Can you work these out from the model? Positions are in its coordinate system, mm. A direction names the side the tool comes from. Round coordinates to 2 decimals unless told otherwise and drop trailing zeros. Loops run counter-clockwise (first coordinate to the right, second up) from the corner with the lowest first, then second, coordinate; pieces in that order, holes last. Notation, with made-up numbers: (76.25, 74.25) -> (116.25, 74.25) arc R26 ccw to (116.25, 111.25) -> close; hole circle Ø5 at (-9.75, -16.5). An arc over 180 degrees is marked (long way). Use a Markdown table: item, result.
Autodesk Inventor part; units mm, degrees
ref_plane "YZ Plane" through (0, 0, 0) normal (1, 0, 0) x (0, 1, 0)
ref_plane "XZ Plane" through (0, 0, 0) normal (0, 1, 0) x (-1, 0, 0)
ref_plane "XY Plane" through (0, 0, 0) normal (0, 0, 1) x (1, 0, 0)
sketch "Sketch1" plane through (0, 0, 0) normal (0, 0, 1) x (1, 0, 0)
  line L0 (0, -70) -> (15, -70)
  line L1 (15, -70) -> (15, 0)
  line L2 (15, 0) -> (0, 0)
  line L3 (0, 0) -> (0, -70)
  line L4 (15, -35) -> (0, -35)
  line L5 (0, -9.5012) -> (15, -9.5012)
  line L6 (15, -9.5012) -> (15, -59.5012)
  line L7 (15, -59.5012) -> (0, -59.5012)
  line L8 (0, -59.5012) -> (0, -9.5012)
  line L9 (0, -9.5012) -> (15, -59.5012) construction
  line L10 (15, -9.5012) -> (0, -59.5012) construction
  line L11 (7.5, -34.5012) -> (7.5349, -35)
  circle A0 centre (7.5349, -35) radius 5.15
  line L12 (0, -70) -> (15, -70)
  line L13 (15, -70) -> (15, -55)
  line L14 (15, -55) -> (0, -55) construction
  line L15 (0, -55) -> (0, -70)
  line L16 (0, 0) -> (15, 0)
  line L17 (15, 0) -> (15, -15)
  line L18 (15, -15) -> (0, -15) construction
  line L19 (0, -15) -> (0, 0)
  line L20 (15, -55) -> (0, -70) construction
  line L21 (0, 0) -> (15, -15) construction
  circle A1 centre (7.5, -62.5) radius 7.5
  circle A2 centre (7.5, -7.5) radius 7.5
  line L22 (0, -59.5012) -> (15, -59.5012)
  line L23 (15, -59.5012) -> (15, -44.5012)
  line L24 (15, -44.5012) -> (0, -44.5012)
  line L25 (0, -44.5012) -> (0, -59.5012)
  line L26 (15, -9.5012) -> (0, -9.5012)
  line L27 (0, -9.5012) -> (0, -24.5012)
  line L28 (0, -24.5012) -> (15, -24.5012)
  line L29 (15, -24.5012) -> (15, -9.5012)
  line L30 (0, -24.5012) -> (15, -9.5012) construction
  line L31 (0, -59.5012) -> (15, -44.5012) construction
  circle A3 centre (7.5, -52.0012) radius 4.05
  circle A4 centre (7.5, -17.0012) radius 4.05
  circle A5 centre (7.5, -62.5) radius 4.05
  circle A6 centre (7.5, -7.5) radius 4.05
  circle A7 centre (7.5, -7.5) radius 4.5
  circle A8 centre (7.5, -62.5) radius 4.5
  point P0 (15, -7.5)
  point P1 (0, -7.5)
  point P2 (0, -62.5)
  point P3 (15, -62.5)
  dimension "d0" = 15
  dimension "d1" = 70
  dimension "d2" = 15
  dimension "d3" = 50
  dimension "d4" = 0.5
  dimension "d5" = 10.3
  dimension "d6" = 15
  dimension "d7" = 15
  dimension "d8" = 15
  dimension "d9" = 15
  dimension "d10" = 15
  dimension "d11" = 15
  dimension "d12" = 15
  dimension "d14" = 8.1
  dimension "d15" = 8.1
  dimension "d16" = 8.1
  dimension "d17" = 8.1
  dimension "d18" = 15
  dimension "d19" = 0
  dimension "d20" = 0
  dimension "d27" = 9
  dimension "d28" = 9
extrude "Extrusion1" add sketch "Sketch1" along normal blind 15 contours A1 L7 A8 | L3 L7 A1 | A1 L7 L1 | L3 L24 L1 L7 A1 A3 | A1 A3 L7 A8 | A8 L7 A5 | L7 A5 A8 | A3 A1 | A1 A3 | L3 L4 A0 L1 L24 | L3 L28 L1 L4 A0 | L3 L5 A2 A4 L1 L28 | L3 A2 L5 | L5 A2 L1 | A2 L5 A7 | L5 A7 A2 A4 | A7 L5 A6 | L5 A6 A7 | A4 A2 | A2 A4
extrude "Extrusion2" add sketch "Sketch1" along normal blind 45 contours A5 L7 | L7 A5 | A6 L5 | L5 A6
extrude "Extrusion3" cut sketch "Sketch1" along normal blind 15 contours A3 A1 | A1 A3 | A4 A2 | A2 A4
extrude "Extrusion4" add sketch "Sketch1" along normal blind 30 contours A8 L7 A5 | L7 A5 A8 | A5 L7 | L7 A5 | A7 L5 A6 | L5 A6 A7 | A6 L5 | L5 A6
fillet "Fillet1" radius 2 8 edges at (7.5, 0, 15) (0, -35, 15) (7.5, -70, 15) (15, -35, 15) (7.5, 0, 0) (0, -35, 0) (7.5, -70, 0) (15, -35, 0)
properties part number "Gear_Holder_2"
1. Will these pins go through, and if not, where does the flat tip stop? pin 1 Ø1.5 at (y, z) = (-62, 36) entering from -X; pin 2 Ø10 at (y, z) = (-18, 18.5) entering from +X; pin 3 Ø9 at (x, y) = (6.5, -27) entering from +Z.
Answer sheet:
| item | result |
|---|---|
| pin 1 | stops at x = 3.45 |
| pin 2 | stops at x = 14.94 |
| pin 3 | stops at z = 15 |
2. I want a section at C-C (z = 22.5). Please give me the cut outline in (x, y), plus the area to 3 significant figures.
Answer sheet:
| item | result |
|---|---|
| outline | circle Ø9 at (7.5, -62.5); circle Ø9 at (7.5, -7.5) |
| area | 127 mm² |
3. I want a section at D-D (x = 9.25). State how many separate pieces and enclosed holes the cut face has, plus the area to 3 significant figures.
Answer sheet:
| item | result |
|---|---|
| separate pieces | 4 |
| enclosed holes | 0 |
| area | 1,140 mm² |
4. I need wall thicknesses on line 1 (Y direction, x = 7.5, z = 8.75); line 2 (Y direction, x = 6.25, z = 4.5); line 3 (X direction, y = -35, z = 4.5). Which ranges of each line are inside material? Lowest first, please.
Answer sheet:
| item | result |
|---|---|
| line 1 | y = -70 to -56.05, -47.95 to -40.15, -29.85 to -21.05, -12.95 to 0 |
| line 2 | y = -69.9 to -55.85, -48.15 to -39.99, -30.01 to -20.85, -13.15 to -0.1 |
| line 3 | x = 0 to 2.38, 12.68 to 15 |
5. If we mould it in two halves opening along X, with no side actions, what happens to faces 1 (the cylindrical face through (0.6, -34.61, 0.57)), 2 (the cylindrical face through (6.62, -48.05, 7.4)), 3 (the flat face through (7, -27, 15))? For each: +X half, -X half, draft (parallel to the pull), parting line (faces both ways), or undercut.
Answer sheet:
| item | result |
|---|---|
| face 1 | -X half |
| face 2 | undercut |
| face 3 | draft |
6. I want a section at A-A (y = -35). Please give me the cut outline in (x, z).
Answer sheet:
| item | result |
|---|---|
| outline | (0, 2) arc R2 ccw to (2, 0) -> (2.38, 0) -> (2.38, 15) -> (2, 15) arc R2 ccw to (0, 13) -> close; (12.68, 0) -> (13, 0) arc R2 ccw to (15, 2) -> (15, 13) arc R2 ccw to (13, 15) -> (12.68, 15) -> close |
7. Which directions (+Z, -Z, +X, -X, +Y, -Y) give clear straight access to the entire face, cutting with the end or side of a thin tool? Please do faces 4 (the cylindrical face through (0.6, -35.39, 14.43)), 5 (the cylindrical face through (6.973, -66.516, 37.395)).
Answer sheet:
| item | result |
|---|---|
| face 4 | +Z, -X, +Y, -Y |
| face 5 | +Z |
8. I want a section at B-B (y = -46.5). Please give me the cut outline in (x, z).
Answer sheet:
| item | result |
|---|---|
| outline | (0, 2) arc R2 ccw to (2, 0) -> (13, 0) arc R2 ccw to (15, 2) -> (15, 13) arc R2 ccw to (13, 15) -> (2, 15) arc R2 ccw to (0, 13) -> close |
